from build123d import *

# Parameters (mm, degrees)
BOSS_EXTRUDE1_DEPTH = 95.25
SKETCH2_R           = 3.175
CUT_EXTRUDE1_DEPTH  = 152.4
SKETCH4_R           = 34.925
SKETCH4_R_2         = 3.81
CUT_EXTRUDE2_DEPTH  = 381
SKETCH5_R           = 3.81
CUT_EXTRUDE3_DEPTH  = 12.7


with BuildPart() as part:
    # Sketch1 → Boss-Extrude1 (new body)
    with BuildSketch(Plane.XY):
        Polygon((0, 0), (0, 381), (3.175, 381), (3.175, 3.175), (473.075, 3.175), (473.075, 0), align=None)
    extrude(amount=BOSS_EXTRUDE1_DEPTH)

    # Sketch2 → Cut-Extrude1 (cut)
    with BuildSketch(Plane(origin=(0, 3.175, 0), x_dir=(1, 0, 0), z_dir=(0, 1, 0))):
        with Locations(Location((190.119, -4.572, 0), (0, 0, 180))):
            Circle(SKETCH2_R)
        with Locations(Location((190.119, -76.2, 0), (0, 0, 180))):
            Circle(SKETCH2_R)
        with Locations(Location((261.747, -4.572, 0), (0, 0, 180))):
            Circle(SKETCH2_R)
        with Locations(Location((261.747, -76.2, 0), (0, 0, 180))):
            Circle(SKETCH2_R)
        with Locations(Location((295.783, -76.2, 0), (0, 0, 180))):
            Circle(SKETCH2_R)
        with Locations(Location((295.783, -4.572, 0), (0, 0, 180))):
            Circle(SKETCH2_R)
        with Locations(Location((367.411, -76.2, 0), (0, 0, 180))):
            Circle(SKETCH2_R)
        with Locations(Location((367.411, -4.572, 0), (0, 0, 180))):
            Circle(SKETCH2_R)
    extrude(amount=-CUT_EXTRUDE1_DEPTH, mode=Mode.SUBTRACT)

    # Sketch4 → Cut-Extrude2 (cut)
    with BuildSketch(Plane.XZ):
        with Locations((225.933, 40.386)):
            Circle(SKETCH4_R)
        with Locations((331.597, 40.386)):
            Circle(SKETCH4_R)
        with Locations((390.525, 19.05)):
            Circle(SKETCH4_R_2)
    extrude(amount=-CUT_EXTRUDE2_DEPTH, mode=Mode.SUBTRACT)

    # Sketch5 → Cut-Extrude3 (cut)
    with BuildSketch(Plane.ZY):
        with Locations((19.05, 349.25)):
            Circle(SKETCH5_R)
    extrude(amount=-CUT_EXTRUDE3_DEPTH, mode=Mode.SUBTRACT)


solid = part.part
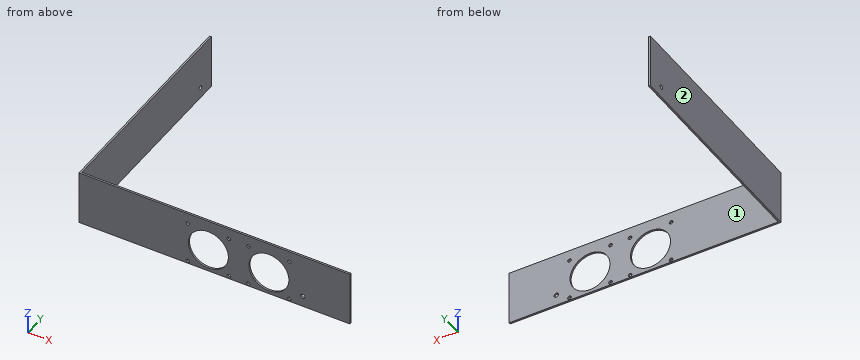
For this review, take the finished solid that the model builds, in its own axes (mm). Face numbers are marked on the shaded views. A direction names the side the tool comes from. Round coordinates to 2 decimals unless told otherwise and drop trailing zeros. Loops run counter-clockwise (first coordinate to the right, second up) from the corner with the lowest first, then second, coordinate; pieces in that order, holes last. Notation, with made-up numbers: (53, 37) - (103, 37) arc R13 cw to (103, 53) - close; hole circle Ø5 at (46.25, -35). An arc over 180 degrees is marked (long way). Use one line per item in the form item = value.
1) We need section B-B on y = 94. Write out the cut boundary in (x, z) (3 decimals), then the cut area to 3 significant figures.
Solutions:
outline = (0, 0) - (3.175, 0) - (3.175, 95.25) - (0, 95.25) - close
area = 302 mm2
2) Tool access review of the marked faces 1 and 2: name each direction out of +Z, -Z, +X, -X, +Y, -Y from which nothing blocks a thin tool from reaching the whole face with its end or side.
Solutions:
face_1 = +Z, -Z, +X, +Y
face_2 = +Z, -Z, -X, +Y, -Y
3) Clearance check with flat-ended pins moving along their axes: P1, Ø10, axis at x = 295.783, z = 76.2, coming from the +Y side (3 decimals); P2, Ø10, axis at y = 349.25, z = 19.05, coming from the +X side (3 decimals). State where each tip first meets the part, or that it passes through.
Solutions:
P1 = 3.175
P2 = 3.175
4) Wall thickness on probe 1 along Y at (x, z) = (0.9, 19.05); probe 2 along Y at (x, z) = (81, 9.5) (3 decimals): over which ranges is each line inside the solid? List them lowest first.
Solutions:
probe_1 = 0 to 345.44, 353.06 to 381
probe_2 = 0 to 3.175
5) We need section A-A on x = 342. Write out the cut boundary in (y, z) (3 decimals).
Solutions:
outline = (0, 0) - (3.175, 0) - (3.175, 7.046) - (0, 7.046) - close; (0, 73.726) - (3.175, 73.726) - (3.175, 95.25) - (0, 95.25) - close
